from build123d import *

# Parameters (mm, degrees)
CUT_EXTRUDE_2_DEPTH = 1
SKETCH_3_R          = 1.5
EXTRUDE_1_DEPTH     = 60


with BuildPart() as part:
    # 草图1 → 旋转1 (revolve)
    with BuildSketch(Plane(origin=(0, 0, 0), x_dir=(0, 0, -1), z_dir=(1, 0, 0))):
        with BuildLine():
            Line((0, 2.250343623), (0, 1))
            Line((0, 1), (0, 0))
            Line((0, 0), (1, 0))
            Line((1, 0), (1, 1))
            Line((1, 1), (1.248177586, 0))
            Line((1.248177586, 0), (1.5, 0))
            Line((1.5, 0), (1.5, 1.5))
            Line((1.5, 1.5), (1.5, 2.8))
            ThreePointArc((1.5, 2.8), (0.701231865, 2.658258964), (0, 2.250343623))
        make_face()
    revolve(axis=Axis((0, 0, 0), (0, 0, -1)))

    # 草图2 → 切除-拉伸2 (cut)
    with BuildSketch(Plane.XY):
        Polygon((0, 1.154700538), (-1, 0.577350269), (-1, -0.577350269), (0, -1.154700538), (1, -0.577350269), (1, 0.577350269), align=None)
    extrude(amount=-CUT_EXTRUDE_2_DEPTH, mode=Mode.SUBTRACT)

    # 草图3 → 凸台-拉伸1 (add)
    with BuildSketch(Plane(origin=(0, 0, -1.5), x_dir=(-1, 0, 0), z_dir=(0, 0, -1))):
        Circle(SKETCH_3_R)
    extrude(amount=EXTRUDE_1_DEPTH)


solid = part.part
Verification items for the finished model (mm, model axes). A direction names the side the tool comes from. Round coordinates to 2 decimals unless told otherwise and drop trailing zeros. Order: outer loops, then holes, each group sorted by start corner. A loop starts at its lowest first (then second) coordinate and runs counter-clockwise, first axis right, second up.
1. Release check for a two-part mould opening along X. For faces 4 (the flat face through (0, 0, -61.5)), 5 (the cylindrical face through (1.5, 0.07, -31.08)), 6 (the flat face through (-0.51, -0.86, -0.49)) record: +X half, -X half, draft (parallel to the pull), parting line (faces both ways), or undercut.
Final values:
face 4: draft
face 5: parting line
face 6: undercut
2. Access from +Z, -Z, +X, -X, +Y, -Y to the whole of each face (thin tool, end or side, straight path). Record for faces 1 (the flat face through (1, 1, 0)), 2 (the flat face through (-0.49, 0.87, -0.49)), 3 (the flat face through (-1.2, -1.2, -1.5)).
Final values:
face 1: +Z, +X, -X, +Y, -Y
face 2: +Z
face 3: -Z
3. Thickness scan on L1, parallel to Z at x = 1.5, y = 1; L2, parallel to Y at x = 0.5, z = -40.5; L3, parallel to X at y = -0.35, z = -2.5. Record the ranges inside material, lowest first.
Final values:
L1: z = -1.5 to 0
L2: y = -1.41 to 1.41
L3: x = -1.46 to 1.46
4. Go/stop test with flat-tipped pins: P1, Ø1, axis at x = -0.5, z = -16, coming from the +Y side; P2, Ø1.5, axis at x = 1, z = -16.5, coming from the -Y side; P3, Ø0.6, axis at x = -0.5, y = 0, coming from the +Z side. Record where each tip stops, or that it passes through.
Final values:
P1: stops at y = 1.5
P2: stops at y = -1.48
P3: stops at z = -1.05
5. Section check A-A on z = -6. Record the cut outline in (x, y), then the cut area to 3 significant figures.
Final values:
outline: circle Ø3 at (0, 0)
area: 7.07 mm2
